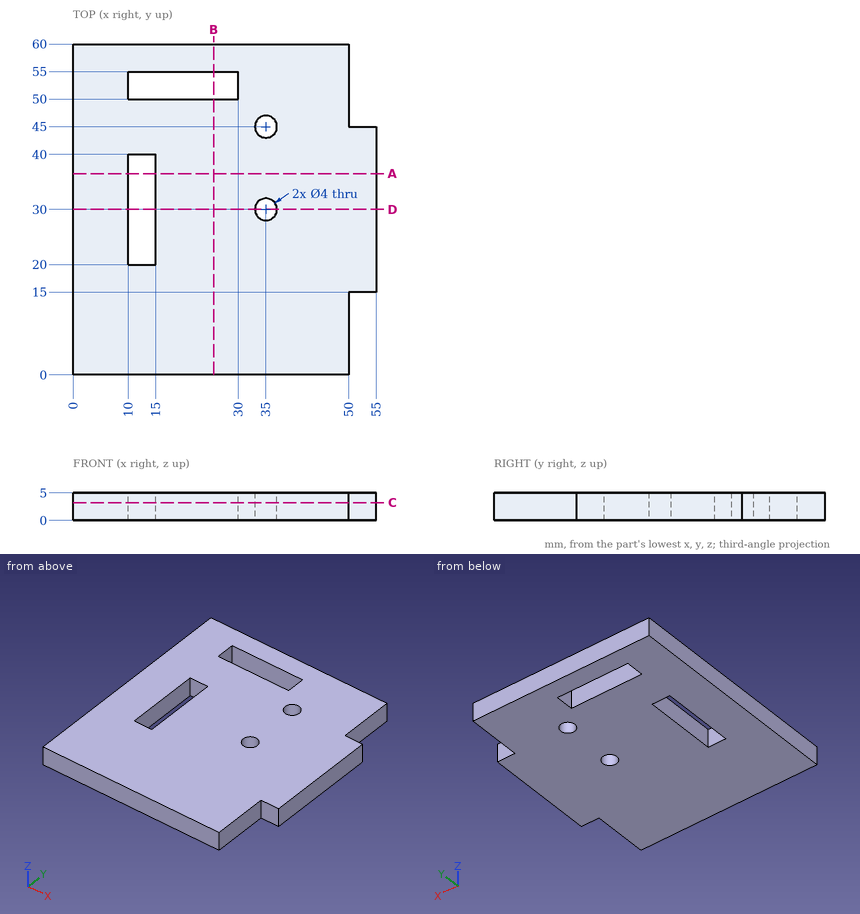
Could you check a few things on this drawing? It's one solid part, dimensions in mm from its lowest x, y, z. Coordinates: 2 decimals unless noted, no trailing zeros. Write each loop counter-clockwise with the first axis right and the second up, starting at its lowest first coordinate (ties: lowest second). Pieces come first, ordered by that corner, then holes. Notation, with made-up numbers: M 18,-37 L 30,-37 A13 ccw 30,-12 Z; hole C 88.5,32.5 d10. An arc over 180 degrees is marked long. Answer as CSV lines item,"result". Start each with the question number.
Q1. Suppose I cut it at D-D, the plane y = 30. List the corners of the cut face in (x, z) for me, then the cut area to 3 significant figures.
Q2. Suppose I cut it at A-A, the plane y = 36.5. List the corners of the cut face in (x, z) for me, then the cut area to 3 significant figures.
Q3. I need wall thicknesses on probe 1 along Y at (x, z) = (35, 1.8); probe 2 along Y at (x, z) = (23.5, 1.15); probe 3 along X at (y, z) = (26.5, 4.35). Which ranges of each line are inside material? Lowest first, please. Write a range as [from, to].
Q4. Suppose I cut it at C-C, the plane z = 3.2. List the corners of the cut face in (x, y) for me, then the cut area to 3 significant figures.
Q5. Will these pins go through, and if not, where does the flat tip stop? pin 1 Ø2.5 at (y, z) = (55, 2.5) entering from +X; pin 2 Ø2 at (x, y) = (28.5, 53) entering from -Z.
Q6. Suppose I cut it at B-B, the plane x = 25.5. List the corners of the cut face in (y, z) for me.
Entries:
1,outline,"M 0,0 L 10,0 L 10,5 L 0,5 Z; M 15,0 L 33,0 L 33,5 L 15,5 Z; M 37,0 L 55,0 L 55,5 L 37,5 Z"
1,area,"230 mm²"
2,outline,"M 0,0 L 10,0 L 10,5 L 0,5 Z; M 15,0 L 55,0 L 55,5 L 15,5 Z"
2,area,"250 mm²"
3,probe 1,"y = [0, 28], [32, 43], [47, 60]"
3,probe 2,"y = [0, 50], [55, 60]"
3,probe 3,"x = [0, 10], [15, 55]"
4,outline,"M 0,0 L 50,0 L 50,15 L 55,15 L 55,45 L 50,45 L 50,60 L 0,60 Z; hole M 10,20 L 15,20 L 15,40 L 10,40 Z; hole M 10,50 L 30,50 L 30,55 L 10,55 Z; hole C 35,30 d4; hole C 35,45 d4"
4,area,"2,920 mm²"
5,pin 1,"stops at x = 50"
5,pin 2,"passes through"
6,outline,"M 0,0 L 50,0 L 50,5 L 0,5 Z; M 55,0 L 60,0 L 60,5 L 55,5 Z"
